```python
from build123d import *

# Parameters (mm, degrees)
SKETCH_1_R      = 22.5
SKETCH_1_R_2    = 1.333333333
EXTRUDE_1_DEPTH = 3
EXTRUDE_2_DEPTH = 60
FILLET_1_R      = 0.5
FILLET_2_R      = 1
FILLET_3_R      = 5


with BuildPart() as part:
    # 草图1 → 凸台-拉伸1 (new body)
    with BuildSketch(Plane(origin=(0, 0, 0), x_dir=(1, 0, 0), z_dir=(0, 1, 0))):
        Circle(SKETCH_1_R)
        with Locations((8.838834765, 8.838834765)):
            Circle(SKETCH_1_R_2, mode=Mode.SUBTRACT)
        with Locations((8.838834765, -8.838834765)):
            Circle(SKETCH_1_R_2, mode=Mode.SUBTRACT)
        with Locations((-8.838834765, -8.838834765)):
            Circle(SKETCH_1_R_2, mode=Mode.SUBTRACT)
        with Locations((-8.838834765, 8.838834765)):
            Circle(SKETCH_1_R_2, mode=Mode.SUBTRACT)
    extrude(amount=EXTRUDE_1_DEPTH)

    # 草图3 → 凸台-拉伸2 (add)
    with BuildSketch(Plane.XZ):
        with BuildLine():
            Line((-23.923076725, 1.92), (23.923076725, 1.92))
            ThreePointArc((23.923076725, 1.92), (24, 0), (23.923076725, -1.92))
            Line((23.923076725, -1.92), (-23.923076725, -1.92))
            ThreePointArc((-23.923076725, -1.92), (-24, 0), (-23.923076725, 1.92))
        make_face()
    extrude(amount=-EXTRUDE_2_DEPTH)

    # 圆角1
    fillet_1_edges = [part.edges().sort_by_distance(p)[0] for p in [
        (-10.172168098, 3, 8.838834765),
        (-10.172168098, 3, -8.838834765),
        (7.505501431, 3, -8.838834765),
        (7.505501431, 3, 8.838834765),
    ]]
    fillet(fillet_1_edges, radius=FILLET_1_R)

    # 圆角2
    fillet_2_edges = [part.edges().sort_by_distance(p)[0] for p in [
        (24, 0, 0),
        (-24, 0, 0),
    ]]
    fillet(fillet_2_edges, radius=FILLET_2_R)

    # 圆角3
    fillet_3_edges = [part.edges().sort_by_distance(p)[0] for p in [
        (-24, 60, 0),
        (24, 60, 0),
    ]]
    fillet(fillet_3_edges, radius=FILLET_3_R)


solid = part.part
```
For this review, take the finished solid that the model builds, in its own axes (mm). A direction names the side the tool comes from. Round coordinates to 2 decimals unless told otherwise and drop trailing zeros. Loops run counter-clockwise (first coordinate to the right, second up) from the corner with the lowest first, then second, coordinate; pieces in that order, holes last.
Q1. Add section C-C on z = 16.5. Write out the cut boundary in (x, y).
Result sheet:
outline: (-15.3, 0) - (15.3, 0) - (15.3, 3) - (-15.3, 3) - close
Q2. Machinability: for faces 1 (the face through (0, 3, 10)), 2 (the face through (-24, 28, 0)), 3 (the face through (0, 3, -10)), which of the approach directions +Z, -Z, +X, -X, +Y, -Y give a long, thin tool a straight path to every point of the face, cutting with its end or side? Answer none if there is none.
Result sheet:
face 1: +Z, +X, -X, +Y
face 2: -X, +Y, -Y
face 3: -Z, +X, -X, +Y
Q3. Add section B-B on x = 3. Write out the cut boundary in (y, z), plus the area to 3 significant figures.
Result sheet:
outline: (0, -22.3) - (3, -22.3) - (3, -1.92) - (60, -1.92) - (60, 1.92) - (3, 1.92) - (3, 22.3) - (0, 22.3) - close
area: 353 mm2
Q4. Insertion check: pin 1 Ø3 at (x, y) = (-8, 36) entering from +Z; pin 2 Ø4 at (x, z) = (-10.5, 13) entering from +Y; pin 3 Ø14.5 at (x, y) = (11.5, 25) entering from -Z. Each pin has a flat end and moves straight along its axis. Give the tip position at first contact, or say it passes through.
Result sheet:
pin 1: stops at z = 1.92
pin 2: stops at y = 3
pin 3: stops at z = -1.92
Q5. To check wall thickness, follow line 1 along Z through (x, y) = (10.5, 10); line 2 along Y through (x, z) = (-8, 13.5); line 3 along X through (y, z) = (18, 1). State the ranges of each line that lie inside material, in increasing order.
Result sheet:
line 1: z = -1.92 to 1.92
line 2: y = 0 to 3
line 3: x = -23.98 to 23.98
Q6. Mouldability with a two-part tool opening along Z and no side actions: class faces 4 (the face through (-9.13, 1.23, 10.14)), 5 (the face through (0, 30, 1.92)), 6 (the face through (0, 30, -1.92)) as +Z half, -Z half, draft (parallel to the pull), parting line (faces both ways), or undercut.
Result sheet:
face 4: undercut
face 5: +Z half
face 6: -Z half
Q7. Add section A-A on y = 7. Write out the cut boundary in (x, z).
Result sheet:
outline: (-23.92, -1.92) - (23.92, -1.92) arc R24 ccw to (23.92, 1.92) - (-23.92, 1.92) arc R24 ccw to start
Q8. Add section D-D on x = 17.5. Write out the cut boundary in (y, z), plus the area to 3 significant figures.
Result sheet:
outline: (0, -14.14) - (3, -14.14) - (3, -1.92) - (60, -1.92) - (60, 1.92) - (3, 1.92) - (3, 14.14) - (0, 14.14) - close
area: 304 mm2
